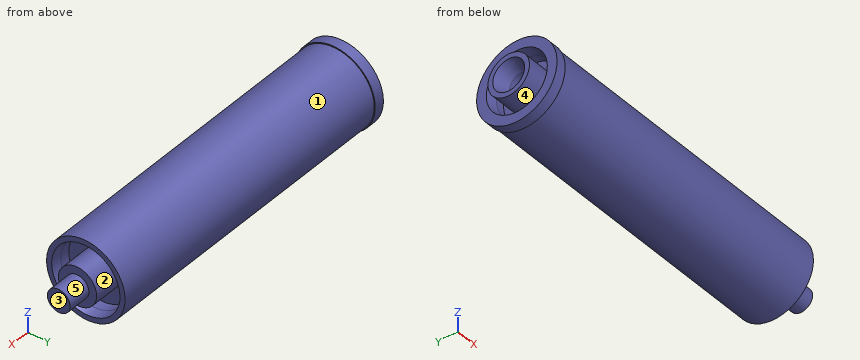
from build123d import *


with BuildPart() as part:
    # Esquisse2 → Révolution7 (revolve)
    with BuildSketch(Plane.XY, mode=Mode.PRIVATE) as r_volution7_sk:
        Polygon((0, 26), (12.7, 26), (36.56741584, 26), (36.56741584, 35.689138439), (25.4, 35.689138439), (12.7, 38.2095), (12.7, 50.419), (25.4, 50.419), (25.4, 49.149), (414.3502, 49.149), (414.3502, 42.820187711), (403.02734835, 40.573126289), (390.454818395, 40.573126289), (390.454818395, 23.9395), (427.3042, 23.9395), (427.3042, 14.2875), (456.5904, 14.2875), (456.5904, 0), (0, 0), align=None)
    revolve(r_volution7_sk.sketch.rotate(Axis((0, 0, 0), (1, 0, 0)), 90), axis=Axis((0, 0, 0), (1, 0, 0)))

    # Esquisse3 → Enlèvement de matière-Révolution1 (revolve, cut)
    with BuildSketch(Plane.XY, mode=Mode.PRIVATE) as enl_vement_de_mati_re_r_volution1_sk:
        Polygon((0, 20), (0, 0), (390.090795287, 0), (390.454818395, 12.957757221), (381.061065959, 12.957757221), (381.061065959, 44.271024873), (65.871878934, 44.271024873), (34.08300614, 14.327580407), (19.08300614, 14.327580407), align=None)
    revolve(enl_vement_de_mati_re_r_volution1_sk.sketch.rotate(Axis((0, 0, 0), (1, 0, 0)), 90), axis=Axis((0, 0, 0), (1, 0, 0)), mode=Mode.SUBTRACT)


solid = part.part
Model file for the job. Use its own axes, mm. Face numbers are marked on the shaded views. A direction names the side the tool comes from. Give positions to 0.01 mm unless a question says otherwise; leave off trailing zeros. Write each loop counter-clockwise with the first axis right and the second up, starting at its lowest first coordinate (ties: lowest second). Pieces come first, ordered by that corner, then holes. Notation, with made-up numbers: M -17.75,58.5 L 12.25,58.5 A27 cw 12.25,80.5 Z; hole C 56.5,3 d6. An arc over 180 degrees is marked long. One line per item, written item: value. Start each with the question number.
Q1. Two-plate mould, pull along Y, no slides. Class the marked faces 1, 2 and 3: +Y half, -Y half, draft (parallel to the pull), parting line (faces both ways), or undercut.
Q2. 3-axis set-ups, long thin cutter, end or side, ignore diameter. For the marked faces 4 and 5: which of +Z, -Z, +X, -X, +Y, -Y reach the whole face in a straight line?
Q3. Drop flat-ended pins along their axis: pin 1 Ø8 at (x, y) = (135, 25) entering from -Z; pin 2 Ø1 at (y, z) = (-9, -2.5) entering from -X; pin 3 Ø10 at (x, z) = (289, -37.5) entering from -Y; pin 4 Ø6 at (y, z) = (-37, 39.5) entering from +X. Give the stop position or say it passes through.
Q4. Saw through at A-A, the plane x = 101.5. Write the cut outline in (y, z), plus the area to 3 significant figures.
Q5. Probe probe 1 along Y at (x, z) = (28.5, 0); probe 2 along Z at (x, y) = (149, -2.5); probe 3 along Y at (x, z) = (260, 0). List the from-to ranges inside material, lowest first. Write a range as [from, to].
Output values:
1. face 1: parting line
1. face 2: undercut
1. face 3: draft
2. face 4: -X
2. face 5: +X
3. pin 1: stops at z = -44.44
3. pin 2: stops at x = 390.34
3. pin 3: stops at y = -36.87
3. pin 4: passes through
4. outline: C 0,0 d98.3; hole C 0,0 d88.54
4. area: 1,430 mm²
5. probe 1: y = [-49.15, -35.69], [-26, -14.33], [14.33, 26], [35.69, 49.15]
5. probe 2: z = [-49.09, -44.2], [44.2, 49.09]
5. probe 3: y = [-49.15, -44.27], [44.27, 49.15]
